Verification items for the finished model (mm, model axes). Face numbers are marked on the shaded views. A direction names the side the tool comes from. Coordinates: 2 decimals unless noted, no trailing zeros. Write each loop counter-clockwise with the first axis right and the second up, starting at its lowest first coordinate (ties: lowest second). Pieces come first, ordered by that corner, then holes. Notation, with made-up numbers: (87.25, 31) -> (105.25, 31) arc R21 cw to (105.25, 35) -> close; hole circle Ø2 at (7.25, -6.5). An arc over 180 degrees is marked (long way). Use CSV: the item, a comma, the result in double quotes.
```python
from build123d import *

# Parameters (mm, degrees)
SKETCH1_W                   = 74.93
SKETCH1_H                   = 101.6
BOSS_EXTRUDE2_DEPTH         = 95.25
CUT_EXTRUDE2_DEPTH          = 145.217712938
CUT_EXTRUDE2_DEPTH_BACK     = 145.217712938
SKETCH4_W                   = 7.62
SKETCH4_H                   = 78.74
BOSS_EXTRUDE3_DEPTH         = 2.54
TAP_DRILL_FOR_1_4_20_TAP1_D = 5.1054
SKETCH9_W                   = 19.05
SKETCH9_H                   = 25.4
CUT_EXTRUDE3_DEPTH          = 73.66
SKETCH10_W                  = 74.93
SKETCH10_H                  = 50.8
CUT_EXTRUDE4_DEPTH          = 63.5
FILLET1_R                   = 12.7


with BuildPart() as part:
    # Sketch1 → Boss-Extrude2 (new body)
    with BuildSketch(Plane.XY):
        Rectangle(SKETCH1_W, SKETCH1_H)
    extrude(amount=-BOSS_EXTRUDE2_DEPTH)

    # Sketch2 → Cut-Extrude2 (cut, two sides: drawn at the far end of the back side and taken through both)
    with BuildSketch(Plane(origin=(0, 50.8, 0), x_dir=(1, 0, 0), z_dir=(0, 1, 0)).offset(-CUT_EXTRUDE2_DEPTH_BACK)):
        with BuildLine():
            Line((-18.542, -230.991823822), (-18.542, 0))
            ThreePointArc((-18.542, 0), (0, 18.542), (18.542, 0))
            Line((18.542, 0), (18.542, -230.991823822))
            Line((18.542, -230.991823822), (18.542, -692.975471465))
            Line((18.542, -692.975471465), (-18.542, -692.975471465))
            Line((-18.542, -692.975471465), (-18.542, -230.991823822))
        make_face()
    extrude(amount=CUT_EXTRUDE2_DEPTH + CUT_EXTRUDE2_DEPTH_BACK, mode=Mode.SUBTRACT)

    # Sketch4 → Boss-Extrude3 (add, symmetric)
    with BuildSketch(Plane(origin=(0, 31.75, 0), x_dir=(1, 0, 0), z_dir=(0, 1, 0))):
        with Locations((0, 55.88)):
            Rectangle(SKETCH4_W, SKETCH4_H)
    extrude(amount=BOSS_EXTRUDE3_DEPTH, both=True)

    # Tap Drill for 1/4-20 Tap1 (through all)
    with Locations(Plane.XY):
        with Locations((-28.7528, 38.1), (28.7528, 38.1), (-28.7528, -38.1), (28.7528, -38.1)):
            Hole(TAP_DRILL_FOR_1_4_20_TAP1_D / 2)

    # Sketch9 → Cut-Extrude3 (cut)
    with BuildSketch(Plane(origin=(0, 0, -95.25), x_dir=(-1, 0, 0), z_dir=(0, 0, -1))):
        with Locations((-27.94, 38.1)):
            Rectangle(SKETCH9_W, SKETCH9_H)
        with Locations((27.94, -38.1)):
            Rectangle(SKETCH9_W, SKETCH9_H)
    extrude(amount=-CUT_EXTRUDE3_DEPTH, mode=Mode.SUBTRACT)

    # Sketch10 → Cut-Extrude4 (cut)
    with BuildSketch(Plane(origin=(0, 0, -95.25), x_dir=(-1, 0, 0), z_dir=(0, 0, -1))):
        Rectangle(SKETCH10_W, SKETCH10_H)
    extrude(amount=-CUT_EXTRUDE4_DEPTH, mode=Mode.SUBTRACT)

    # Fillet1
    fillet1_edges = [part.edges().sort_by_distance(p)[0] for p in [
        (-9.525, 25.4, -31.75),
        (9.525, -25.4, -31.75),
    ]]
    fillet(fillet1_edges, radius=FILLET1_R)


solid = part.part
```
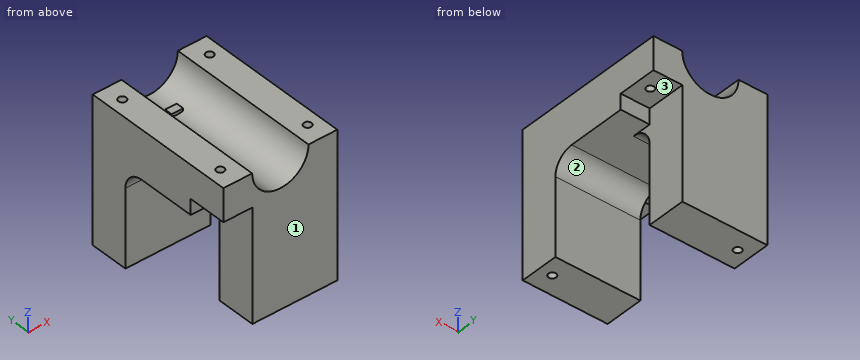
1) Cross-section at C-C (x = 0). Record the boundary of the cut face in (y, z), plus the area to 3 significant figures.
Return value:
outline,"(-50.8, -95.25) -> (-25.4, -95.25) -> (-25.4, -44.45) arc R12.7 cw to (-12.7, -31.75) -> (12.7, -31.75) arc R12.7 cw to (25.4, -44.45) -> (25.4, -95.25) -> (50.8, -95.25) -> (50.8, -18.54) -> (34.29, -18.54) -> (34.29, -16.51) -> (29.21, -16.51) -> (29.21, -18.54) -> (-50.8, -18.54) -> close"
area,"4,650 mm2"
2) Cross-section at B-B (y = -38.1). Give the number of separate pieces and of enclosed holes in the cut face, plus the area to 3 significant figures.
Return value:
separate pieces,"3"
enclosed holes,"0"
area,"4,600 mm2"
3) Scan lines: L1, parallel to Y at x = -8, z = -89; L2, parallel to X at y = 38, z = -13 (3 decimals); L3, parallel to X at y = -28, z = -59 (3 decimals). Record each from-to range of solid material in increasing order.
Return value:
L1,"-50.8 to -25.4, 25.4 to 50.8"
L2,"-37.465 to -31.304, -26.202 to -13.221, 13.221 to 26.202, 31.304 to 37.465"
L3,"-18.415 to 37.465"
4) Cross-section at A-A (z = -51.5). Record the boundary of the cut face in (x, y) (1 decimal).
Return value:
outline,"(-37.5, 25.4) -> (18.4, 25.4) -> (18.4, 50.8) -> (-37.5, 50.8) -> close; (-18.4, -50.8) -> (37.5, -50.8) -> (37.5, -25.4) -> (-18.4, -25.4) -> close; hole circle Ø5.1 at (-28.8, 38.1); hole circle Ø5.1 at (28.8, -38.1)"
5) Cross-section at D-D (z = -37). Record the boundary of the cut face in (x, y) (1 decimal), plus the area to 3 significant figures.
Return value:
outline,"(-37.5, 23) -> (18.4, 23) -> (18.4, 50.8) -> (-37.5, 50.8) -> close; (-18.4, -50.8) -> (37.5, -50.8) -> (37.5, -23) -> (-18.4, -23) -> close; hole circle Ø5.1 at (-28.8, 38.1); hole circle Ø5.1 at (28.8, -38.1)"
area,"3,070 mm2"
6) Set-up check for the marked faces 1, 2 and 3: record each of +Z, -Z, +X, -X, +Y, -Y from which the full face is reachable in a straight line by a thin tool's end or side.
Return value:
face 1,"+Z, -Z, +X, -X, -Y"
face 2,"-Z, +X, -X"
face 3,"-Z, +X, +Y"
7) Gauge pin test, flat ends, axial feed: pin 1 (19 mm diameter, centred on y = 33, z = -62.5, fed in from +X) (3 decimals); pin 2 (9.5 mm diameter, centred on x = -28.5, y = -39, fed in from -Z); pin 3 (8 mm diameter, centred on x = -4, y = -13.5, fed in from -Z). Record the tip position at first contact, or that the pin passes through.
Return value:
pin 1,"x = 18.415"
pin 2,"z = -21.59"
pin 3,"z = -32.69"
